The listing builds one solid part. Answer for the finished solid, in the listing's coordinates (mm). Coordinates: 2 decimals unless noted, no trailing zeros. Write each loop counter-clockwise with the first axis right and the second up, starting at its lowest first coordinate (ties: lowest second). Pieces come first, ordered by that corner, then holes.
(1) The part is cut by section B-B on z = 2.25. Determine the outline of the cut face in (x, y), plus the area to 3 significant figures.
(2) For a pull along Y with two mould halves and no side action, classify faces 1 (the cylindrical face through (-5.38, -16.57, 10.85)), 2 (the flat face through (-1, -10, 0)), 3 (the cylindrical face through (47.69, 15.02, 10.85)) as +Y half, -Y half, draft (parallel to the pull), parting line (faces both ways), or undercut.
(3) The part is cut by section D-D on y = 20. Determine the outline of the cut face in (x, z).
(4) The part is cut by section A-A on x = 0. Determine the outline of the cut face in (y, z).
(5) Given P1, Ø5, axis at y = -5, z = 9, coming from the +X side; P2, Ø1.5, axis at y = 5, z = 19.5, coming from the +X side; P3, Ø2, axis at x = 15, z = 14.5, coming from the -Y side, each flat-ended and moving along its own axis, determine where each tip first touches the part or whether it passes through.
(6) Straight lines are drawn through the part: line 1 (Y direction, x = 0, z = 20.5); line 2 (Y direction, x = -26, z = 6.25); line 3 (Y direction, x = -6, z = 1.5). For each, find the intervals that lie inside material, in ascending order.
(7) The part is cut by section C-C on x = 27. Determine the outline of the cut face in (y, z), plus the area to 3 significant figures.
from build123d import *

# Parameters (mm, degrees)
ESQUISSE1_R             = 50
BOSS_EXTRU_1_DEPTH      = 22
ESQUISSE2_R             = 2.5
ENL_V_MAT_EXTRU_1_DEPTH = 7
ENL_V_START             = -15
ENL_V_MAT_EXTRU_3_DEPTH = 15
ESQUISSE4_R             = 10
ENL_V_MAT_EXTRU_5_DEPTH = 22
ESQUISSE5_R             = 10
ENL_V_MAT_EXTRU_6_DEPTH = 22
ESQUISSE6_R             = 10
ENL_V_MAT_EXTRU_7_DEPTH = 22
ESQUISSE7_R             = 10
ENL_V_MAT_EXTRU_8_DEPTH = 22


with BuildPart() as part:
    # Esquisse1 → Boss.-Extru.1 (new body)
    with BuildSketch(Plane.XY):
        Circle(ESQUISSE1_R)
    extrude(amount=BOSS_EXTRU_1_DEPTH)

    # Esquisse2 → Enlèv. mat.-Extru.1 (cut)
    with BuildSketch(Plane.XY.offset(22)):
        Circle(ESQUISSE2_R)
    extrude(amount=-ENL_V_MAT_EXTRU_1_DEPTH, mode=Mode.SUBTRACT)

    # Esquisse3 → Enlèv. mat.-Extru.3 (cut)
    with BuildSketch(Plane(origin=(0, 0, 0), x_dir=(-1, 0, 0), z_dir=(0, 0, -1)).offset(ENL_V_START)):
        with BuildLine():
            ThreePointArc((2.5, 0), (0.559569372, 2.436571796), (-2.249505694, 1.09074476))
            Line((-2.249505694, 1.09074476), (-2.366104086, -0.807187373))
            ThreePointArc((-2.366104086, -0.807187373), (0.409108657, -2.466298868), (2.5, 0))
        make_face()
    extrude(amount=ENL_V_MAT_EXTRU_3_DEPTH, mode=Mode.SUBTRACT)

    # Esquisse4 → Enlèv. mat.-Extru.5 (cut)
    with BuildSketch(Plane(origin=(0, 0, 0), x_dir=(-1, 0, 0), z_dir=(0, 0, -1))):
        with Locations((0, 25)):
            Circle(ESQUISSE4_R)
    extrude(amount=-ENL_V_MAT_EXTRU_5_DEPTH, mode=Mode.SUBTRACT)

    # Esquisse5 → Enlèv. mat.-Extru.6 (cut)
    with BuildSketch(Plane(origin=(0, 0, 0), x_dir=(-1, 0, 0), z_dir=(0, 0, -1))):
        with Locations((25, 0)):
            Circle(ESQUISSE5_R)
    extrude(amount=-ENL_V_MAT_EXTRU_6_DEPTH, mode=Mode.SUBTRACT)

    # Esquisse6 → Enlèv. mat.-Extru.7 (cut)
    with BuildSketch(Plane(origin=(0, 0, 0), x_dir=(-1, 0, 0), z_dir=(0, 0, -1))):
        with Locations((0, -25)):
            Circle(ESQUISSE6_R)
    extrude(amount=-ENL_V_MAT_EXTRU_7_DEPTH, mode=Mode.SUBTRACT)

    # Esquisse7 → Enlèv. mat.-Extru.8 (cut)
    with BuildSketch(Plane(origin=(0, 0, 0), x_dir=(-1, 0, 0), z_dir=(0, 0, -1))):
        with Locations((-25, 0)):
            Circle(ESQUISSE7_R)
    extrude(amount=-ENL_V_MAT_EXTRU_8_DEPTH, mode=Mode.SUBTRACT)


solid = part.part
Model answer:
1. outline: circle Ø100 at (0, 0); hole circle Ø20 at (-25, 0); hole circle Ø20 at (0, -25); hole circle Ø20 at (0, 25); hole (2.25, 1.09) arc R2.5 ccw (long way) to (2.37, -0.81) - close; hole circle Ø20 at (25, 0)
1. area: 6,580 mm2
2. face 1: undercut
2. face 2: draft
2. face 3: parting line
3. outline: (-45.83, 0) - (-8.66, 0) - (-8.66, 22) - (-45.83, 22) - close; (8.66, 0) - (45.83, 0) - (45.83, 22) - (8.66, 22) - close
4. outline: (-50, 0) - (-35, 0) - (-35, 22) - (-50, 22) - close; (-15, 0) - (-2.5, 0) - (-2.5, 22) - (-15, 22) - close; (2.5, 0) - (15, 0) - (15, 22) - (2.5, 22) - close; (35, 0) - (50, 0) - (50, 22) - (35, 22) - close
5. P1: stops at x = 49.94
5. P2: stops at x = 49.82
5. P3: stops at y = -48
6. line 1: y = -50 to -35, -15 to -2.5, 2.5 to 15, 35 to 50
6. line 2: y = -42.71 to -9.95, 9.95 to 42.71
6. line 3: y = -49.64 to -33, -17 to 17, 33 to 49.64
7. outline: (-42.08, 0) - (-9.8, 0) - (-9.8, 22) - (-42.08, 22) - close; (9.8, 0) - (42.08, 0) - (42.08, 22) - (9.8, 22) - close
7. area: 1,420 mm2
